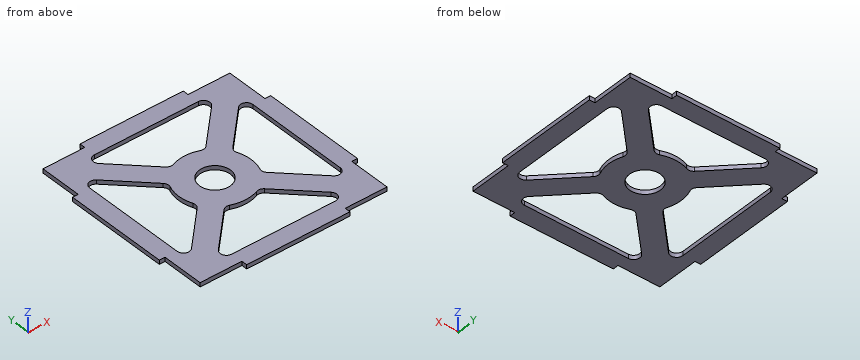
from build123d import *

# Parameters (mm, degrees)
F1_DEPTH = 2
F2_R     = 7.5
F3_DEPTH = 25
F4_R     = 3


with BuildPart() as f1:
    # F0 (on Top) → F1 (new body)
    with BuildSketch(Plane.XY):
        Polygon((25, 45.25), (25, 48), (-25, 48), (-25, 45.25), (-45.25, 45.25), (-45.25, 25), (-48, 25), (-48, -25), (-45.25, -25), (-45.25, -45.25), (-25, -45.25), (-25, -48), (25, -48), (25, -45.25), (45.25, -45.25), (45.25, -25), (48, -25), (48, 25), (45.25, 25), (45.25, 45.25), align=None)
    extrude(amount=F1_DEPTH)

    # F2 (on face) → F3 (cut)
    with BuildSketch(Plane.XY.offset(2)):
        with BuildLine():
            ThreePointArc((-15.394075, -8.323007), (-17.5, 0), (-15.394075, 8.323007))
            Line((-15.394075, 8.323007), (-39.5, 32.428932))
            Line((-39.5, 32.428932), (-39.5, -32.428932))
            Line((-39.5, -32.428932), (-15.394075, -8.323007))
        make_face()
        with BuildLine():
            Line((-32.428932, 39.5), (-8.323007, 15.394075))
            ThreePointArc((-8.323007, 15.394075), (0, 17.5), (8.323007, 15.394075))
            Line((8.323007, 15.394075), (32.428932, 39.5))
            Line((32.428932, 39.5), (-32.428932, 39.5))
        make_face()
        Circle(F2_R)
        with BuildLine():
            ThreePointArc((15.394075, 8.323007), (17.5, 0), (15.394075, -8.323007))
            Line((15.394075, -8.323007), (39.5, -32.428932))
            Line((39.5, -32.428932), (39.5, 32.428932))
            Line((39.5, 32.428932), (15.394075, 8.323007))
        make_face()
        with BuildLine():
            Line((-32.428932, -39.5), (32.428932, -39.5))
            Line((32.428932, -39.5), (8.323007, -15.394075))
            ThreePointArc((8.323007, -15.394075), (0, -17.5), (-8.323007, -15.394075))
            Line((-8.323007, -15.394075), (-32.428932, -39.5))
        make_face()
    extrude(amount=-F3_DEPTH, mode=Mode.SUBTRACT)

    # F4
    f4_edges = [f1.edges().sort_by_distance(p)[0] for p in [
        (-39.5, 32.428932, 1),
        (-15.394075, -8.323007, 1),
        (-15.394075, 8.323007, 1),
        (8.323007, 15.394075, 1),
        (-8.323007, 15.394075, 1),
        (-32.428932, -39.5, 1),
        (15.394075, -8.323007, 1),
        (15.394075, 8.323007, 1),
        (39.5, -32.428932, 1),
        (39.5, 32.428932, 1),
        (32.428932, 39.5, 1),
        (32.428932, -39.5, 1),
        (-39.5, -32.428932, 1),
        (-32.428932, 39.5, 1),
        (-8.323007, -15.394075, 1),
        (8.323007, -15.394075, 1),
    ]]
    fillet(f4_edges, radius=F4_R)


solid = f1.part
Can you work these out from the model? Positions are in its coordinate system, mm. Round coordinates to 2 decimals unless told otherwise and drop trailing zeros. Loops run counter-clockwise (first coordinate to the right, second up) from the corner with the lowest first, then second, coordinate; pieces in that order, holes last. Notation, with made-up numbers: (-7.5, -12) - (33.5, -12) arc R9 cw to (33.5, -6) - close; hole circle Ø4 at (13, 23). An arc over 180 degrees is marked (long way). Answer in a Markdown table with one row per item. Add a question column.
Q1. For pin 1 Ø1 at (x, z) = (-47, 1) entering from -Y; pin 2 Ø1 at (x, z) = (-31.5, 0.5) entering from -Y; pin 3 Ø0.6 at (y, z) = (37, 1) entering from -X, each with a flat end and sliding along its axis, tell me the tip position at first contact or that it passes through.
Q2. I want a section at B-B on x = 37. List the corners of the cut face in (y, z) for me.
Q3. I want a section at D-D on x = -2. List the corners of the cut face in (y, z) for me, and give its area (3 significant figures).
Q4. I want a section at C-C on y = 33. List the corners of the cut face in (x, z) for me, and give its area (3 significant figures).
Q5. I need wall thicknesses on L1, parallel to X at y = -0.5, z = 0.75; L2, parallel to X at y = 15.5, z = 0.85; L3, parallel to Y at x = -24, z = 1.95. Which ranges of each line are inside material? Lowest first, please.
Q6. I want a section at A-A on y = 0. List the corners of the cut face in (x, z) for me.
A:
| question | item | result |
|---|---|---|
| 1 | pin 1 | y = -25 |
| 1 | pin 2 | y = -45.25 |
| 1 | pin 3 | x = -45.25 |
| 2 | outline | (-45.25, 0) - (-28.14, 0) - (-28.14, 2) - (-45.25, 2) - close; (28.14, 0) - (45.25, 0) - (45.25, 2) - (28.14, 2) - close |
| 3 | outline | (-48, 0) - (-39.5, 0) - (-39.5, 2) - (-48, 2) - close; (-17.39, 0) - (-7.23, 0) - (-7.23, 2) - (-17.39, 2) - close; (7.23, 0) - (17.39, 0) - (17.39, 2) - (7.23, 2) - close; (39.5, 0) - (48, 0) - (48, 2) - (39.5, 2) - close |
| 3 | area | 74.6 mm^2 |
| 4 | outline | (-45.25, 0) - (-25.93, 0) - (-25.93, 2) - (-45.25, 2) - close; (25.93, 0) - (45.25, 0) - (45.25, 2) - (25.93, 2) - close |
| 4 | area | 77.3 mm^2 |
| 5 | L1 | -48 to -39.5, -17.49 to -7.48, 7.48 to 17.49, 39.5 to 48 |
| 5 | L2 | -48 to -39.5, -22.57 to 22.57, 39.5 to 48 |
| 5 | L3 | -48 to -39.5, -31.07 to -16.93, 16.93 to 31.07, 39.5 to 48 |
| 6 | outline | (-48, 0) - (-39.5, 0) - (-39.5, 2) - (-48, 2) - close; (-17.5, 0) - (-7.5, 0) - (-7.5, 2) - (-17.5, 2) - close; (7.5, 0) - (17.5, 0) - (17.5, 2) - (7.5, 2) - close; (39.5, 0) - (48, 0) - (48, 2) - (39.5, 2) - close |
